```python
from build123d import *

# Parameters (mm, degrees)
SKETCH3_W           = 47.5
SKETCH3_H           = 22.5
BOSS_EXTRUDE1_DEPTH = 2
SKETCH56_R          = 0.99762119
CUT_EXTRUDE1_DEPTH  = 10
SKETCH53_R          = 0.995230863
CUT_EXTRUDE2_DEPTH  = 10
SKETCH52_R          = 1
CUT_EXTRUDE3_DEPTH  = 10
SKETCH57_R          = 1
CUT_EXTRUDE4_DEPTH  = 10
SKETCH74_W          = 12.004185621
SKETCH74_H          = 3.004883548
CUT_EXTRUDE6_DEPTH  = 10
SKETCH79_W          = 47.5
SKETCH79_H          = 2
BOSS_EXTRUDE2_DEPTH = 21.190075336
FILLET6_R           = 2


with BuildPart() as part:
    # Sketch3 → Boss-Extrude1 (new body)
    with BuildSketch(Plane(origin=(0, 0, 0), x_dir=(1, 0, 0), z_dir=(0, 1, 0))):
        with Locations((-56.111912524, -4.514800621)):
            Rectangle(SKETCH3_W, SKETCH3_H)
    extrude(amount=BOSS_EXTRUDE1_DEPTH)

    # Sketch56 → Cut-Extrude1 (cut)
    with BuildSketch(Plane(origin=(0, 0, 0), x_dir=(-1, 0, 0), z_dir=(0, -1, 0))):
        with Locations(Location((34.326389274, -13.765097561, 0), (0, 0, 90))):
            Circle(SKETCH56_R)
    extrude(amount=-CUT_EXTRUDE1_DEPTH, mode=Mode.SUBTRACT)

    # Sketch53 → Cut-Extrude2 (cut)
    with BuildSketch(Plane(origin=(0.004388193, 0, 0), x_dir=(-1, 0, 0), z_dir=(0, -1, 0))):
        with Locations(Location((34.328904029, 4.735389548, 0), (0, 0, 90))):
            Circle(SKETCH53_R)
    extrude(amount=-CUT_EXTRUDE2_DEPTH, mode=Mode.SUBTRACT)

    # Sketch52 → Cut-Extrude3 (cut)
    with BuildSketch(Plane(origin=(0, 0, -0.040736422), x_dir=(1, 0, 0), z_dir=(0, -1, 0))):
        with Locations(Location((-77.82393232, -4.694462956, 0), (0, 0, 270))):
            Circle(SKETCH52_R)
    extrude(amount=-CUT_EXTRUDE3_DEPTH, mode=Mode.SUBTRACT)

    # Sketch57 → Cut-Extrude4 (cut)
    with BuildSketch(Plane.XZ):
        with Locations(Location((-77.826389274, 13.764800621, 0), (0, 0, 270))):
            Circle(SKETCH57_R)
    extrude(amount=-CUT_EXTRUDE4_DEPTH, mode=Mode.SUBTRACT)

    # Sketch74 → Cut-Extrude6 (cut)
    with BuildSketch(Plane(origin=(0, 2, 0), x_dir=(1, 0, 0), z_dir=(0, 1, 0))):
        with Locations((-56.07183951, 5.232757605)):
            Rectangle(SKETCH74_W, SKETCH74_H)
    extrude(amount=-CUT_EXTRUDE6_DEPTH, mode=Mode.SUBTRACT)

    # Sketch79 → Boss-Extrude2 (add)
    with BuildSketch(Plane(origin=(0, 0, 0), x_dir=(1, 0, 0), z_dir=(0, 1, 0))):
        with Locations((-56.111912524, -16.764800621)):
            Rectangle(SKETCH79_W, SKETCH79_H)
    extrude(amount=BOSS_EXTRUDE2_DEPTH)

    # Fillet6
    # the kernel refuses this fillet: 2 mm, written as the material it adds along each edge
    with BuildSketch(Plane(origin=(-32.361912524, 2, 15.764800621), x_dir=(0, 1, 0), z_dir=(-1, 0, 0))) as fillet6_piece_1_section:
        with BuildLine():
            CenterArc((FILLET6_R, FILLET6_R), FILLET6_R, 180, 90)
            Line((0, FILLET6_R), (0, 0))
            Line((0, 0), (FILLET6_R, 0))
        make_face()
    fillet6_piece_1 = extrude(amount=47.5, mode=Mode.PRIVATE)
    fillet6_piece_1 = fillet6_piece_1 - Plane(origin=(-34.326389274, 2.455648449, 13.765097561), x_dir=(0, 0, -1), z_dir=(0, -1, 0)) * Cylinder(0.99762119, 103, mode=Mode.PRIVATE)
    fillet6_piece_1 = fillet6_piece_1 - Plane(origin=(-77.826389274, 2.455648449, 13.764800621), x_dir=(0, 0, -1), z_dir=(0, -1, 0)) * Cylinder(1, 103, mode=Mode.PRIVATE)
    add(fillet6_piece_1)


solid = part.part
```
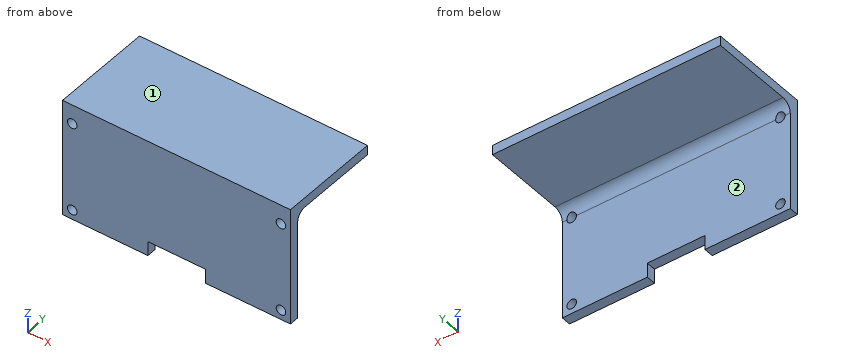
Input: part model. Units: mm. Frame: model coordinates. Face numbers are marked on the shaded views. A direction names the side the tool comes from. Give positions to 0.01 mm unless a question says otherwise; leave off trailing zeros. Order: outer loops, then holes, each group sorted by start corner. A loop starts at its lowest first (then second) coordinate and runs counter-clockwise, first axis right, second up. Notation, with made-up numbers: M 58.5,11 L 91.5,11 A21 cw 91.5,46 Z; hole C 35,-12 d4. An arc over 180 degrees is marked long. Return JSON: item names as keys, results as strings.
1) Access query for the marked faces 1 and 2. Directions: +Z, -Z, +X, -X, +Y, -Y. A direction counts if a zero-diameter tool reaches every point of the face in a straight line with its end or side. Return the directions, or none.
Taken from the geometry:
{"face 1": "+Z, +X, -X, +Y, -Y", "face 2": "-Z, +X, -X, +Y"}
2) Section query D-D on x = -60. Output: boundary loops of the cut face in (y, z).
Taken from the geometry:
{"outline": "M 0,-3.73 L 2,-3.73 L 2,13.76 A2 cw 4,15.76 L 21.19,15.76 L 21.19,17.76 L 0,17.76 Z"}
3) Section query A-A on x = -70. Output: boundary loops of the cut face in (y, z).
Taken from the geometry:
{"outline": "M 0,-6.74 L 2,-6.74 L 2,13.76 A2 cw 4,15.76 L 21.19,15.76 L 21.19,17.76 L 0,17.76 Z"}
4) Contact query for flat-ended pins moving along their axis: pin 1 (8 mm diameter, centred on x = -53.5, y = 14.5, fed in from -Z); pin 2 (2.5 mm diameter, centred on x = -77.83, z = 13.76, fed in from +Y); pin 3 (1.6 mm diameter, centred on x = -58.5, y = 1, fed in from -Z); pin 4 (1.2 mm diameter, centred on x = -34.32, z = -4.74, fed in from +Y) (1 decimal). Output: stop coordinate, or through.
Taken from the geometry:
{"pin 1": "stops at z = 15.76", "pin 2": "stops at y = 2.43", "pin 3": "stops at z = -3.73", "pin 4": "passes through"}
5) Line query: L1, parallel to Y at x = -35, z = -0.25; L2, parallel to Z at x = -63, y = 12.5; L3, parallel to Z at x = -67, y = 3. Output: solid intervals per line, ascending. Write a range as [from, to].
Taken from the geometry:
{"L1": "y = [0, 2]", "L2": "z = [15.76, 17.76]", "L3": "z = [15.5, 17.76]"}
6) Section query B-B on y = 1.5. Output: boundary loops of the cut face in (x, z), and give its area (3 significant figures).
Taken from the geometry:
{"outline": "M -79.86,-6.74 L -62.07,-6.74 L -62.07,-3.73 L -50.07,-3.73 L -50.07,-6.74 L -32.36,-6.74 L -32.36,17.76 L -79.86,17.76 Z; hole C -77.83,13.76 d2; hole C -77.82,-4.74 d2; hole C -34.32,-4.74 d1.99; hole C -34.33,13.77 d2", "area": "1,120 mm2"}
7) Section query C-C on y = 11. Output: boundary loops of the cut face in (x, z).
Taken from the geometry:
{"outline": "M -79.86,15.76 L -32.36,15.76 L -32.36,17.76 L -79.86,17.76 Z"}
